Read the model definition and answer for the solid it produces. Units are mm, in the model's axes. Face numbers are marked on the shaded views. A direction names the side the tool comes from. Round coordinates to 2 decimals unless told otherwise and drop trailing zeros. Write each loop counter-clockwise with the first axis right and the second up, starting at its lowest first coordinate (ties: lowest second). Pieces come first, ordered by that corner, then holes. Notation, with made-up numbers: (-12.5, -13) - (23.5, -13) arc R21 cw to (23.5, 16) - close; hole circle Ø10 at (17, 76). An arc over 180 degrees is marked (long way). Answer as CSV lines item,"result". Start each with the question number.
1) Find section B-B on z = 0. Determine the outline of the cut face in (x, y), then the cut area to 3 significant figures.
2) Which of the six approach directions +Z, -Z, +X, -X, +Y, -Y give full straight-line access (tool end or side, diameter ignored) to the marked faces 1 and 2?
3) Consider line 1 along X through (y, z) = (-3, 0); line 2 along Y through (x, z) = (-6, 19); line 3 along Z through (x, y) = (-16, 50.5). Determine where each line is inside the solid, lowest interval first.
4) Each of these flat-tipped pins is pushed along its axis until it touches: pin 1 (1.6 mm diameter, centred on x = 15, y = 26, fed in from -Z); pin 2 (1.2 mm diameter, centred on x = -20.5, y = 40.5, fed in from -Z); pin 3 (10 mm diameter, centred on x = 16, z = -1, fed in from -Y); pin 4 (1.2 mm diameter, centred on x = 20, y = 58.5, fed in from -Z). Where does it stop, or does it pass through?
5) Find section A-A on x = 0. Determine the outline of the cut face in (y, z).
6) Find section C-C on z = 11. Determine the outline of the cut face in (x, y), then the cut area to 3 significant figures.
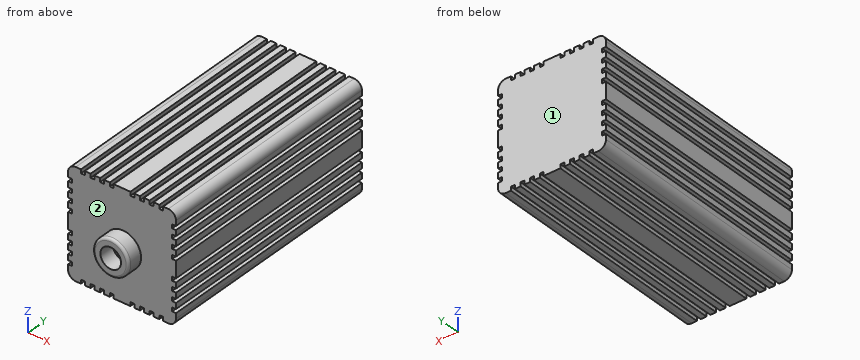
from build123d import *

# Parameters (mm, degrees)
BOSS_EXTRU_1_DEPTH = 90
ESQUISSE2_R        = 7
ESQUISSE2_R_2      = 4
BOSS_EXTRU_2_DEPTH = 6
CONG_1_R           = 1


with BuildPart() as part:
    # Esquisse1 → Boss.-Extru.1 (new body)
    with BuildSketch(Plane(origin=(0, 0, 0), x_dir=(1, 0, 0), z_dir=(0, 1, 0))):
        with BuildLine():
            Line((-19.909227763, -17.432297172), (-21.409227763, -17.432297172))
            Line((-21.409227763, -17.432297172), (-21.409227763, -19.432297172))
            ThreePointArc((-21.409227763, -19.432297172), (-20.530548107, -21.553617516), (-18.409227763, -22.432297172))
            Line((-18.409227763, -22.432297172), (-16.409227763, -22.432297172))
            Line((-16.409227763, -22.432297172), (-16.409227763, -20.932297172))
            Line((-16.409227763, -20.932297172), (-14.909227763, -20.932297172))
            Line((-14.909227763, -20.932297172), (-14.909227763, -22.432297172))
            Line((-14.909227763, -22.432297172), (-12.659227763, -22.432297172))
            Line((-12.659227763, -22.432297172), (-12.659227763, -20.932297172))
            Line((-12.659227763, -20.932297172), (-11.159227763, -20.932297172))
            Line((-11.159227763, -20.932297172), (-11.159227763, -22.432297172))
            Line((-11.159227763, -22.432297172), (-8.909227763, -22.432297172))
            Line((-8.909227763, -22.432297172), (-8.909227763, -20.932297172))
            Line((-8.909227763, -20.932297172), (-7.409227763, -20.932297172))
            Line((-7.409227763, -20.932297172), (-7.409227763, -22.432297172))
            Line((-7.409227763, -22.432297172), (-5.159227763, -22.432297172))
            Line((-5.159227763, -22.432297172), (-5.159227763, -20.932297172))
            Line((-5.159227763, -20.932297172), (-3.659227763, -20.932297172))
            Line((-3.659227763, -20.932297172), (-3.659227763, -22.432297172))
            Line((-3.659227763, -22.432297172), (2.840772237, -22.432297172))
            Line((2.840772237, -22.432297172), (2.840772237, -20.932297172))
            Line((2.840772237, -20.932297172), (4.340772237, -20.932297172))
            Line((4.340772237, -20.932297172), (4.340772237, -22.432297172))
            Line((4.340772237, -22.432297172), (6.590772237, -22.432297172))
            Line((6.590772237, -22.432297172), (6.590772237, -20.932297172))
            Line((6.590772237, -20.932297172), (8.090772237, -20.932297172))
            Line((8.090772237, -20.932297172), (8.090772237, -22.432297172))
            Line((8.090772237, -22.432297172), (10.340772237, -22.432297172))
            Line((10.340772237, -22.432297172), (10.340772237, -20.932297172))
            Line((10.340772237, -20.932297172), (11.840772237, -20.932297172))
            Line((11.840772237, -20.932297172), (11.840772237, -22.432297172))
            Line((11.840772237, -22.432297172), (14.090772237, -22.432297172))
            Line((14.090772237, -22.432297172), (14.090772237, -20.932297172))
            Line((14.090772237, -20.932297172), (15.590772237, -20.932297172))
            Line((15.590772237, -20.932297172), (15.590772237, -22.432297172))
            Line((15.590772237, -22.432297172), (17.590772237, -22.432297172))
            ThreePointArc((17.590772237, -22.432297172), (19.71209258, -21.553617516), (20.590772237, -19.432297172))
            Line((20.590772237, -19.432297172), (20.590772237, -17.432297172))
            Line((20.590772237, -17.432297172), (19.090772237, -17.432297172))
            Line((19.090772237, -17.432297172), (19.090772237, -15.932297172))
            Line((19.090772237, -15.932297172), (20.590772237, -15.932297172))
            Line((20.590772237, -15.932297172), (20.590772237, -13.682297172))
            Line((20.590772237, -13.682297172), (19.090772237, -13.682297172))
            Line((19.090772237, -13.682297172), (19.090772237, -12.182297172))
            Line((19.090772237, -12.182297172), (20.590772237, -12.182297172))
            Line((20.590772237, -12.182297172), (20.590772237, -9.932297172))
            Line((20.590772237, -9.932297172), (19.090772237, -9.932297172))
            Line((19.090772237, -9.932297172), (19.090772237, -8.432297172))
            Line((19.090772237, -8.432297172), (20.590772237, -8.432297172))
            Line((20.590772237, -8.432297172), (20.590772237, -6.182297172))
            Line((20.590772237, -6.182297172), (19.090772237, -6.182297172))
            Line((19.090772237, -6.182297172), (19.090772237, -4.682297172))
            Line((19.090772237, -4.682297172), (20.590772237, -4.682297172))
            Line((20.590772237, -4.682297172), (20.590772237, 1.817702828))
            Line((20.590772237, 1.817702828), (19.090772237, 1.817702828))
            Line((19.090772237, 1.817702828), (19.090772237, 3.317702828))
            Line((19.090772237, 3.317702828), (20.590772237, 3.317702828))
            Line((20.590772237, 3.317702828), (20.590772237, 5.567702828))
            Line((20.590772237, 5.567702828), (19.090772237, 5.567702828))
            Line((19.090772237, 5.567702828), (19.090772237, 7.067702828))
            Line((19.090772237, 7.067702828), (20.590772237, 7.067702828))
            Line((20.590772237, 7.067702828), (20.590772237, 9.317702828))
            Line((20.590772237, 9.317702828), (19.090772237, 9.317702828))
            Line((19.090772237, 9.317702828), (19.090772237, 10.817702828))
            Line((19.090772237, 10.817702828), (20.590772237, 10.817702828))
            Line((20.590772237, 10.817702828), (20.590772237, 13.067702828))
            Line((20.590772237, 13.067702828), (19.090772237, 13.067702828))
            Line((19.090772237, 13.067702828), (19.090772237, 14.567702828))
            Line((19.090772237, 14.567702828), (20.590772237, 14.567702828))
            Line((20.590772237, 14.567702828), (20.590772237, 16.567702828))
            ThreePointArc((20.590772237, 16.567702828), (19.71209258, 18.689023171), (17.590772237, 19.567702828))
            Line((17.590772237, 19.567702828), (15.590772237, 19.567702828))
            Line((15.590772237, 19.567702828), (15.590772237, 18.067702828))
            Line((15.590772237, 18.067702828), (14.090772237, 18.067702828))
            Line((14.090772237, 18.067702828), (14.090772237, 19.567702828))
            Line((14.090772237, 19.567702828), (11.840772237, 19.567702828))
            Line((11.840772237, 19.567702828), (11.840772237, 18.067702828))
            Line((11.840772237, 18.067702828), (10.340772237, 18.067702828))
            Line((10.340772237, 18.067702828), (10.340772237, 19.567702828))
            Line((10.340772237, 19.567702828), (8.090772237, 19.567702828))
            Line((8.090772237, 19.567702828), (8.090772237, 18.067702828))
            Line((8.090772237, 18.067702828), (6.590772237, 18.067702828))
            Line((6.590772237, 18.067702828), (6.590772237, 19.567702828))
            Line((6.590772237, 19.567702828), (4.340772237, 19.567702828))
            Line((4.340772237, 19.567702828), (4.340772237, 18.067702828))
            Line((4.340772237, 18.067702828), (2.840772237, 18.067702828))
            Line((2.840772237, 18.067702828), (2.840772237, 19.567702828))
            Line((2.840772237, 19.567702828), (-3.659227763, 19.567702828))
            Line((-3.659227763, 19.567702828), (-3.659227763, 18.067702828))
            Line((-3.659227763, 18.067702828), (-5.159227763, 18.067702828))
            Line((-5.159227763, 18.067702828), (-5.159227763, 19.567702828))
            Line((-5.159227763, 19.567702828), (-7.409227763, 19.567702828))
            Line((-7.409227763, 19.567702828), (-7.409227763, 18.067702828))
            Line((-7.409227763, 18.067702828), (-8.909227763, 18.067702828))
            Line((-8.909227763, 18.067702828), (-8.909227763, 19.567702828))
            Line((-8.909227763, 19.567702828), (-11.159227763, 19.567702828))
            Line((-11.159227763, 19.567702828), (-11.159227763, 18.067702828))
            Line((-11.159227763, 18.067702828), (-12.659227763, 18.067702828))
            Line((-12.659227763, 18.067702828), (-12.659227763, 19.567702828))
            Line((-12.659227763, 19.567702828), (-14.909227763, 19.567702828))
            Line((-14.909227763, 19.567702828), (-14.909227763, 18.067702828))
            Line((-14.909227763, 18.067702828), (-16.409227763, 18.067702828))
            Line((-16.409227763, 18.067702828), (-16.409227763, 19.567702828))
            Line((-16.409227763, 19.567702828), (-18.409227763, 19.567702828))
            ThreePointArc((-18.409227763, 19.567702828), (-20.530548107, 18.689023171), (-21.409227763, 16.567702828))
            Line((-21.409227763, 16.567702828), (-21.409227763, 14.567702828))
            Line((-21.409227763, 14.567702828), (-19.909227763, 14.567702828))
            Line((-19.909227763, 14.567702828), (-19.909227763, 13.067702828))
            Line((-19.909227763, 13.067702828), (-21.409227763, 13.067702828))
            Line((-21.409227763, 13.067702828), (-21.409227763, 10.817702828))
            Line((-21.409227763, 10.817702828), (-19.909227763, 10.817702828))
            Line((-19.909227763, 10.817702828), (-19.909227763, 9.317702828))
            Line((-19.909227763, 9.317702828), (-21.409227763, 9.317702828))
            Line((-21.409227763, 9.317702828), (-21.409227763, 7.067702828))
            Line((-21.409227763, 7.067702828), (-19.909227763, 7.067702828))
            Line((-19.909227763, 7.067702828), (-19.909227763, 5.567702828))
            Line((-19.909227763, 5.567702828), (-21.409227763, 5.567702828))
            Line((-21.409227763, 5.567702828), (-21.409227763, 3.317702828))
            Line((-21.409227763, 3.317702828), (-19.909227763, 3.317702828))
            Line((-19.909227763, 3.317702828), (-19.909227763, 1.817702828))
            Line((-19.909227763, 1.817702828), (-21.409227763, 1.817702828))
            Line((-21.409227763, 1.817702828), (-21.409227763, -4.682297172))
            Line((-21.409227763, -4.682297172), (-19.909227763, -4.682297172))
            Line((-19.909227763, -4.682297172), (-19.909227763, -6.182297172))
            Line((-19.909227763, -6.182297172), (-21.409227763, -6.182297172))
            Line((-21.409227763, -6.182297172), (-21.409227763, -8.432297172))
            Line((-21.409227763, -8.432297172), (-19.909227763, -8.432297172))
            Line((-19.909227763, -8.432297172), (-19.909227763, -9.932297172))
            Line((-19.909227763, -9.932297172), (-21.409227763, -9.932297172))
            Line((-21.409227763, -9.932297172), (-21.409227763, -12.182297172))
            Line((-21.409227763, -12.182297172), (-19.909227763, -12.182297172))
            Line((-19.909227763, -12.182297172), (-19.909227763, -13.682297172))
            Line((-19.909227763, -13.682297172), (-21.409227763, -13.682297172))
            Line((-21.409227763, -13.682297172), (-21.409227763, -15.932297172))
            Line((-21.409227763, -15.932297172), (-19.909227763, -15.932297172))
            Line((-19.909227763, -15.932297172), (-19.909227763, -17.432297172))
        make_face()
    extrude(amount=BOSS_EXTRU_1_DEPTH)

    # Esquisse2 → Boss.-Extru.2 (add)
    with BuildSketch(Plane.XZ):
        with Locations(Location((0, 0, 0), (0, 0, 90))):
            Circle(ESQUISSE2_R)
        with Locations(Location((0, 0, 0), (0, 0, 270))):
            Circle(ESQUISSE2_R_2, mode=Mode.SUBTRACT)
    extrude(amount=BOSS_EXTRU_2_DEPTH)

    # Congé1
    cong_1_edges = [part.edges().sort_by_distance(p)[0] for p in [
        (0, -6, -7),
    ]]
    fillet(cong_1_edges, radius=CONG_1_R)


solid = part.part
Check values:
1,outline,"(-21.41, 0) - (-7, 0) - (-7, -5) arc R1 ccw to (-6, -6) - (-4, -6) - (-4, 0) - (4, 0) - (4, -6) - (6, -6) arc R1 ccw to (7, -5) - (7, 0) - (20.59, 0) - (20.59, 90) - (-21.41, 90) - close"
1,area,"3,820 mm^2"
2,face 1,"+Z, -Z, +X, -X, +Y"
2,face 2,"-Y"
3,line 1,"x = -7 to -4, 4 to 7"
3,line 2,"y = 0 to 90"
3,line 3,"z = -18.07 to 20.93"
4,pin 1,"stops at z = -19.57"
4,pin 2,"stops at z = -19.17"
4,pin 3,"stops at y = 0"
4,pin 4,"stops at z = -18.96"
5,outline,"(-6, -6) arc R1 ccw to (-5, -7) - (0, -7) - (0, -19.57) - (90, -19.57) - (90, 22.43) - (0, 22.43) - (0, 7) - (-5, 7) arc R1 ccw to (-6, 6) - (-6, 4) - (0, 4) - (0, -4) - (-6, -4) - close"
6,outline,"(-21.41, 0) - (20.59, 0) - (20.59, 90) - (-21.41, 90) - close"
6,area,"3,780 mm^2"
